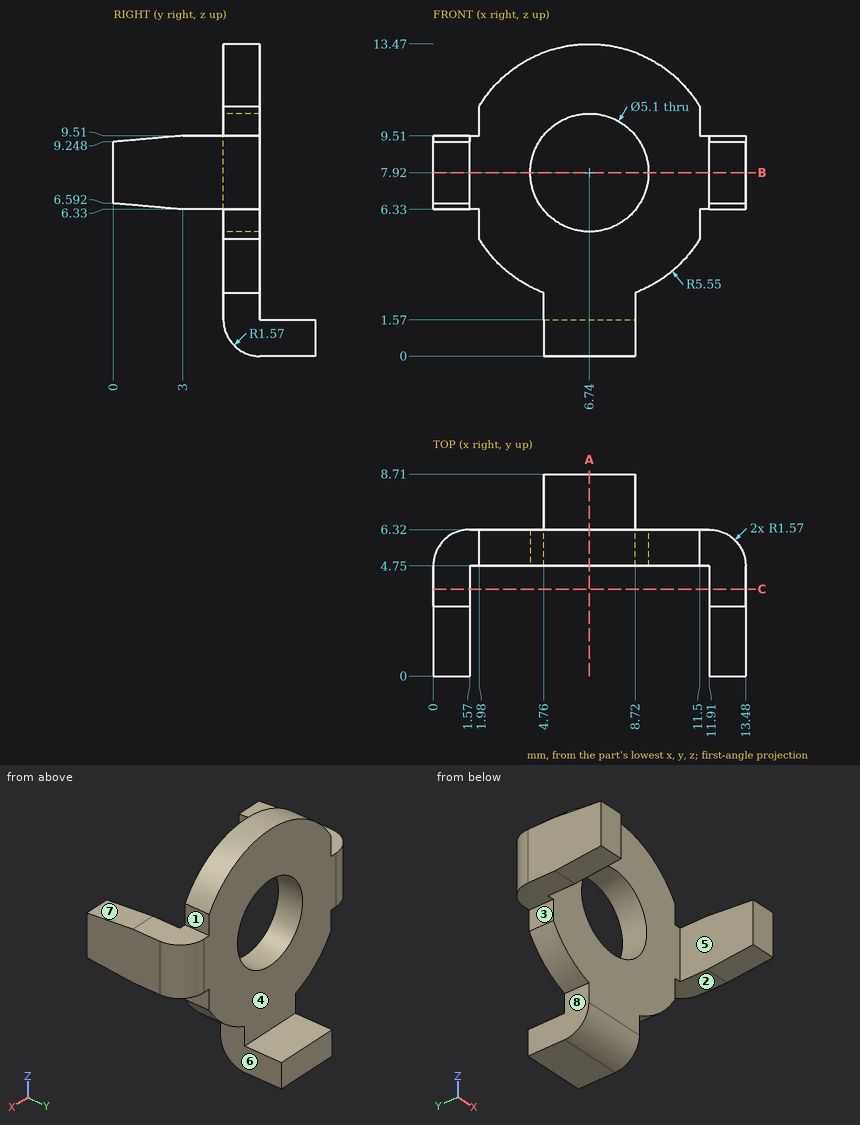
Check sheet for the drawn part. Datum: minimum x, y, z corner. Units: mm. A direction names the side the tool comes from. Round coordinates to 2 decimals unless told otherwise and drop trailing zeros. Order: outer loops, then holes, each group sorted by start corner. A loop starts at its lowest first (then second) coordinate and runs counter-clockwise, first axis right, second up. Notation, with made-up numbers: (45.25, -5) -> (89.25, -5) arc R30 ccw to (89.25, 33) -> close; hole circle Ø3 at (86.25, -35.75). An arc over 180 degrees is marked (long way). Return JSON: item names as keys, results as strings. Group by question number.
Q1. Gauge pin test, flat ends, axial feed: pin 1 (1.4 mm diameter, centred on y = 5.5, z = 6, fed in from -X) (1 decimal); pin 2 (5 mm diameter, centred on x = 4.5, z = 9, fed in from -Y); pin 3 (1.4 mm diameter, centred on y = 5.5, z = 10.5, fed in from +X). Record the tip position at first contact, or that the pin passes through.
Q2. Section check B-B, the plane z = 7.92. Record the boundary of the cut face in (x, y).
Q3. Material ranges on probe 1 along X at (y, z) = (3.5, 9.25); probe 2 along X at (y, z) = (5.25, 2.25); probe 3 along Z at (x, y) = (6.74, 5.15) (1 decimal), recorded low to high. Write a range as from..to.
Q4. Section check C-C, the plane y = 3.75. Record the boundary of the cut face in (x, z).
Q5. Release check for a two-part mould opening along X. For the marked faces 5, 6, 7 and 8 record: released by +X, released by -X, zero draft, split by the parting line, or undercut.
Q6. Tool access check on the marked faces 1, 2, 3 and 4. Record the directions out of +Z, -Z, +X, -X, +Y, -Y that give a thin tool (end or side, any length) a straight path to the whole face; none if there is none.
Q7. Section check A-A, the plane x = 6.74. Record the boundary of the cut face in (y, z).
Numbers:
{
 "1": {"pin 1": "x = 0", "pin 2": "y = 4.75", "pin 3": "x = 11.5"},
 "2": {"outline": "(0, 0) -> (1.57, 0) -> (1.57, 4.75) -> (4.19, 4.75) -> (4.19, 6.32) -> (1.57, 6.32) arc R1.57 ccw to (0, 4.75) -> close; (9.29, 4.75) -> (11.91, 4.75) -> (11.91, 0) -> (13.48, 0) -> (13.48, 4.75) arc R1.57 ccw to (11.91, 6.32) -> (9.29, 6.32) -> close"},
 "3": {"probe 1": "0..1.57, 11.91..13.48", "probe 2": "4.76..8.72", "probe 3": "0.5..5.4, 10.5..13.5"},
 "4": {"outline": "(0, 6.33) -> (1.57, 6.33) -> (1.57, 9.51) -> (0, 9.51) -> close; (11.91, 6.33) -> (13.48, 6.33) -> (13.48, 9.51) -> (11.91, 9.51) -> close"},
 "5": {"face 5": "undercut", "face 6": "released by +X", "face 7": "zero draft", "face 8": "released by -X"},
 "6": {"face 1": "+Z, +X, +Y, -Y", "face 2": "-Z, +X, +Y, -Y", "face 3": "-Z, -X, +Y, -Y", "face 4": "+Z, +X, -X, +Y"},
 "7": {"outline": "(4.75, 1.57) arc R1.57 ccw to (6.32, 0) -> (8.71, 0) -> (8.71, 1.57) -> (6.32, 1.57) -> (6.32, 5.37) -> (4.75, 5.37) -> close; (4.75, 10.47) -> (6.32, 10.47) -> (6.32, 13.47) -> (4.75, 13.47) -> close"}
}
